from build123d import *

# Parameters (mm, degrees)
IZIM1_R                     = 1.5
Y_KSEKLIK_EKSTR_ZYON1_DEPTH = 2
Y_KSEKLIK_EKSTR_ZYON2_DEPTH = 38.08
KAT_Y_D_N_T_R1_START        = 2
KAT_Y_D_N_T_R1_OUTLINE_W    = 38.08
KAT_Y_D_N_T_R1_OUTLINE_H    = 11
KAT_Y_D_N_T_R1_DEPTH        = 6
KENAR_START                 = -15.383826754
KENAR_EKME1_DEPTH           = 38.08
PAH2_SIZE                   = 1
KES_EKSTR_ZYON1_START       = -1
KES_EKSTR_ZYON1_DEPTH       = 1
KES_EKSTR_ZYON2_DEPTH       = 1


# Read off the part's stored shape, not the designer's step: Katıyı-Dönüştür1, Kenar Çekme1
with BuildPart() as part:
    # Çizim1 → Yükseklik-Ekstrüzyon1 (new body)
    with BuildSketch(Plane(origin=(0, 0, 0), x_dir=(1, 0, 0), z_dir=(0, 1, 0))):
        with BuildLine():
            Line((-12.383826754, -1.619350185), (-2.804796795, -1.619350185))
            Line((-2.804796795, -1.619350185), (19.696173246, -1.619350185))
            ThreePointArc((19.696173246, -1.619350185), (21.81749359, -2.498029841), (22.696173246, -4.619350185))
            Line((22.696173246, -4.619350185), (22.696173246, -24.732233603))
            Line((22.696173246, -24.732233603), (22.696173246, -29.619350185))
            Line((22.696173246, -29.619350185), (-15.383826754, -29.619350185))
            Line((-15.383826754, -29.619350185), (-15.383826754, -12.116060357))
            Line((-15.383826754, -12.116060357), (-15.383826754, -4.619350185))
            ThreePointArc((-15.383826754, -4.619350185), (-14.505147098, -2.498029841), (-12.383826754, -1.619350185))
        make_face()
        with Locations(Location((3.656173246, -8.619350185, 0), (0, 0, 270))):
            Circle(IZIM1_R, mode=Mode.SUBTRACT)
        with Locations(Location((-10.425087976, -5.646549714, 0), (0, 0, 270))):
            Circle(IZIM1_R, mode=Mode.SUBTRACT)
        with Locations(Location((17.737434468, -5.646549714, 0), (0, 0, 90))):
            Circle(IZIM1_R, mode=Mode.SUBTRACT)
    extrude(amount=Y_KSEKLIK_EKSTR_ZYON1_DEPTH)

    # Çizim2 → Yükseklik-Ekstrüzyon2 (add)
    with BuildSketch(Plane(origin=(22.696173246, 0, 0), x_dir=(0, 0, -1), z_dir=(1, 0, 0))):
        with BuildLine():
            Line((-19.271126131, 3), (-17.130193592, 3))
            ThreePointArc((-17.130193592, 3), (-23.452666681, 7.16227766), (-21.003176939, 0))
            Line((-21.003176939, 0), (-17.003176939, 0))
            Line((-17.003176939, 0), (-17.003176939, 2))
            Line((-17.003176939, 2), (-21.003176939, 2))
            ThreePointArc((-21.003176939, 2), (-22.003176939, 5.732050808), (-19.271126131, 3))
        make_face()
    extrude(amount=-Y_KSEKLIK_EKSTR_ZYON2_DEPTH)

    # Katıyı-Dönüştür1 outline → Katıyı-Dönüştür1 (cut)
    with BuildSketch(Plane(origin=(0, 0, 0), x_dir=(1, 0, 0), z_dir=(0, 1, 0)).offset(KAT_Y_D_N_T_R1_START)):
        with Locations((3.656173246, -21.5)):
            Rectangle(KAT_Y_D_N_T_R1_OUTLINE_W, KAT_Y_D_N_T_R1_OUTLINE_H)
    extrude(amount=KAT_Y_D_N_T_R1_DEPTH, mode=Mode.SUBTRACT)

    # Kenar Çekme1 outline → Kenar Çekme1 (add)
    with BuildSketch(Plane.YZ.offset(KENAR_START)):
        with BuildLine():
            Line((3.448725288, 27.696826793), (2.897450577, 25.774303401))
            ThreePointArc((2.897450577, 25.774303401), (7.19454204, 32.026610277), (0, 29.619350185))
            Line((0, 29.619350185), (2, 29.619350185))
            ThreePointArc((2, 29.619350185), (5.59727102, 30.822980231), (3.448725288, 27.696826793))
        make_face()
    extrude(amount=KENAR_EKME1_DEPTH)

    # Pah2
    pah2_edges = [part.edges().sort_by_distance(p)[0] for p in [
        (-10.425087976, 2, 4.146549714),
        (3.656173246, 2, 7.119350185),
        (17.737434468, 2, 7.146549714),
    ]]
    chamfer(pah2_edges, length=PAH2_SIZE)

    # Çizim11 → Kes-Ekstrüzyon1 (cut)
    with BuildSketch(Plane(origin=(22.696173246, 0, 0), x_dir=(0, 0, -1), z_dir=(1, 0, 0)).offset(KES_EKSTR_ZYON1_START)):
        with BuildLine():
            Line((-25.774303401, 2.897450577), (-25.774303401, 0))
            Line((-25.774303401, 0), (-29.619350185, 0))
            ThreePointArc((-29.619350185, 0), (-32.026610277, 7.19454204), (-25.774303401, 2.897450577))
        make_face()
    extrude(amount=KES_EKSTR_ZYON1_DEPTH, mode=Mode.SUBTRACT)

    # Çizim12 → Kes-Ekstrüzyon2 (cut)
    with BuildSketch(Plane.ZY.offset(15.383826754)):
        with BuildLine():
            Line((25.774303401, 2.897450577), (25.774303401, 0))
            Line((25.774303401, 0), (29.619350185, 0))
            ThreePointArc((29.619350185, 0), (32.026610277, 7.19454204), (25.774303401, 2.897450577))
        make_face()
    extrude(amount=-KES_EKSTR_ZYON2_DEPTH, mode=Mode.SUBTRACT)


solid = part.part
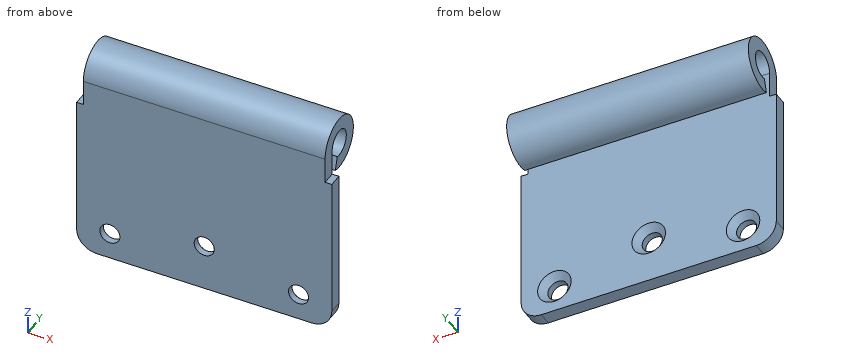
For this review, take the finished solid that the model builds, in its own axes (mm). Coordinates: 2 decimals unless noted, no trailing zeros. Loops run counter-clockwise (first coordinate to the right, second up) from the corner with the lowest first, then second, coordinate; pieces in that order, holes last. Notation, with made-up numbers: (42.25, 30) - (48.25, 30) arc R12 ccw to (48.25, 40) - close; hole circle Ø4 at (37.5, 16). An arc over 180 degrees is marked (long way). Return JSON: item names as keys, results as strings.
Item 1: Take a section at A-A (y = 4). Give the boundary of the cut face in (x, z).
Determined:
{"outline": "(-14.38, 25.62) - (21.7, 25.62) - (21.7, 27.62) - (-14.38, 27.62) - close; (-14.38, 31.62) - (21.7, 31.62) - (21.7, 33.62) - (-14.38, 33.62) - close"}
Item 2: For line 1 (Z direction, x = 4.5, y = 4); line 2 (Y direction, x = 2, z = 11); line 3 (Y direction, x = -2.5, z = 30.5), list the stretches that pass through material, from the lowest coordinate up.
Determined:
{"line 1": "z = 25.62 to 27.62, 31.62 to 33.62", "line 2": "y = 0 to 2", "line 3": "y = 0.1 to 2.2, 5.8 to 7.9"}
Item 3: Take a section at C-C (z = 16.5). Give the boundary of the cut face in (x, y).
Determined:
{"outline": "(-15.38, 0) - (22.7, 0) - (22.7, 2) - (-15.38, 2) - close"}
Item 4: Take a section at D-D (y = 6.5). Give the boundary of the cut face in (x, z).
Determined:
{"outline": "(-14.38, 26.5) - (21.7, 26.5) - (21.7, 32.74) - (-14.38, 32.74) - close"}
Item 5: Insertion check: pin 1 (2 mm diameter, centred on x = -6.5, y = 2, fed in from +Z); pin 2 (4.5 mm diameter, centred on y = 4, z = 29.62, fed in from -X); pin 3 (12 mm diameter, centred on x = 8.5, z = 18, fed in from +Y). Each pin has a flat end and moves straight along its axis. Give the tip position at first contact, or say it passes through.
Determined:
{"pin 1": "stops at z = 33.49", "pin 2": "stops at x = -14.38", "pin 3": "stops at y = 2"}
Item 6: Take a section at B-B (x = -5). Give the boundary of the cut face in (y, z), then the cut area to 4 significant figures.
Determined:
{"outline": "(0, 1.62) - (2, 1.62) - (2, 29.62) arc R2 cw (long way) to (3.45, 27.7) - (2.9, 25.77) arc R4 ccw (long way) to (0, 29.62) - close", "area": "85.95 mm2"}
